Can you work these out from the model? Positions are in its coordinate system, mm. Face numbers are marked on the shaded views. A direction names the side the tool comes from. Coordinates: 2 decimals unless noted, no trailing zeros. Write each loop counter-clockwise with the first axis right and the second up, starting at its lowest first coordinate (ties: lowest second). Pieces come first, ordered by that corner, then holes. Notation, with made-up numbers: M 0,25.25 L 11,25.25 A6 ccw 11,29.25 Z; hole C -0.5,-2 d3. An arc over 180 degrees is marked long. Use one line per item in the form item = value. Start each with the question number.
Autodesk Fusion 360 part; units mm, degrees
sketch "Sketch1" plane through (0, 0, 0) normal (1, 0, 0) x (0, 1, 0)
  line L0 (0, 0) -> (-25.4, 0)
  line L1 (-25.4, 0) -> (-25.4, 43.18)
  line L2 (-25.4, 43.18) -> (-19.05, 43.18)
  line L3 (0, 0) -> (0, 43.18)
  line L4 (0, 43.18) -> (-6.35, 43.18)
  line L5 (-6.35, 43.18) -> (-6.35, 17.78)
  line L6 (-19.05, 43.18) -> (-19.05, 17.7768)
  line L7 (-19.05, 17.7768) -> (-6.35, 17.78)
  circle A0 centre (-12.7, 7.62) radius 5.08
  dimension "d1" = 25.4
  dimension "d2" = 43.18
  dimension "d3" = 6.35
  dimension "d5" = 25.4
  dimension "d6" = 10.16
  dimension "d7" = 12.7
  dimension "d8" = 7.62
  dimension "d10" = 6.35
  dimension "d11" = 12.7
  dimension "d12" = 43.18
extrude "Extrude1" add sketch "Sketch1" along normal blind 25.4
sketch "Sketch2" plane through (25.4, 0, 0) normal (1, 0, 0) x (0, 1, 0)
  circle A0 centre (-12.7, 7.62) radius 5.08
  line L0 (0, 0) -> (0, 43.18)
  line L1 (0, 43.18) -> (-6.35, 43.18)
  line L2 (-6.35, 43.18) -> (-6.35, 17.78)
  line L3 (-6.35, 17.78) -> (-19.05, 17.7768)
  line L4 (-19.05, 17.7768) -> (-19.05, 43.18)
  line L5 (-19.05, 43.18) -> (-25.4, 43.18)
  line L6 (-25.4, 43.18) -> (-25.4, 0)
  line L7 (-25.4, 0) -> (0, 0)
  line L8 (-25.4, 0) -> (0, 0)
  line L9 (0, 0) -> (0, 16.51)
  line L10 (0, 16.51) -> (-25.4, 16.51)
  line L11 (-25.4, 16.51) -> (-25.4, 0)
  dimension "d28" = 16.51
extrude "Extrude2" cut sketch "Sketch2" against normal blind 6.3551 contours L0 L6 L7 L8 L9 L10 L11
sketch "Sketch3" plane through (0, 0, 0) normal (-1, 0, 0) x (0, -1, 0)
  circle A0 centre (12.7, 7.62) radius 5.08
  line L0 (0, 43.18) -> (0, 0)
  line L1 (0, 0) -> (25.4, 0)
  line L2 (25.4, 0) -> (25.4, 43.18)
  line L3 (25.4, 43.18) -> (19.05, 43.18)
  line L4 (19.05, 43.18) -> (19.05, 17.7768)
  line L5 (19.05, 17.7768) -> (6.35, 17.78)
  line L6 (6.35, 17.78) -> (6.35, 43.18)
  line L7 (6.35, 43.18) -> (0, 43.18)
  line L8 (0, 0) -> (25.4, 0)
  line L9 (25.4, 0) -> (25.4, 16.51)
  line L10 (25.4, 16.51) -> (0, 16.51)
  line L11 (0, 16.51) -> (0, 0)
  dimension "d29" = 16.51
extrude "Extrude3" cut sketch "Sketch3" against normal blind 6.3551 contours L0 L1 L2 L8 L9 L10 L11
sketch "Sketch4" plane through (0, -25.4, 0) normal (0, -1, 0) x (1, 0, 0)
  line L0 (6.3551, 16.51) -> (6.3551, 0)
  line L1 (6.3551, 0) -> (19.0449, 0)
  line L2 (19.0449, 0) -> (19.0449, 16.51)
  line L3 (19.0449, 16.51) -> (25.4, 16.51)
  line L4 (25.4, 16.51) -> (25.4, 43.18)
  line L5 (25.4, 43.18) -> (0, 43.18)
  line L6 (0, 43.18) -> (0, 16.51)
  line L7 (0, 16.51) -> (6.3551, 16.51)
  line L8 (0, 43.18) -> (25.4422, 43.18)
  line L9 (25.4422, 43.18) -> (25.4422, 17.78)
  line L10 (25.4422, 17.78) -> (0, 17.78)
  line L11 (0, 17.78) -> (0, 43.18)
  circle A0 centre (12.7, 25.4) radius 2.54
  circle A1 centre (12.7, 35.56) radius 5.08
  dimension "d19" = 25.4
  dimension "d20" = 5.08
  dimension "d22" = 12.7
  dimension "d23" = 10.16
  dimension "d24" = 7.62
  dimension "d25" = 12.7
  dimension "d47" = 10.16
extrude "Extrude4" cut sketch "Sketch4" against normal blind 40.64 contours A0 | A1
fillet "Fillet1" radius 12.7 2 edges at (12.7, -25.4, 0) (12.7, 0, 0)
chamfer "Chamfer1" distance 6.0452 angle 50 2 edges at (25.4, -22.225, 43.18) (25.4, -3.175, 43.18) measured on face at (8.4667, -23.2833, 43.18) measured on face at (8.4667, -2.1167, 43.18)
chamfer "Chamfer2" distance 4.572 angle 20 1 edges at (0, -3.175, 43.18) measured on face at (12.9032, -2.1167, 43.18)
chamfer "Chamfer3" distance 4.572 angle 20 1 edges at (0, -22.225, 43.18) measured on face at (12.9032, -23.2833, 43.18)
sketch "Sketch5" plane through (0, -25.4, 0) normal (0, -1, 0) x (1, 0, 0)
  line L0 (4.572, 43.18) -> (0, 41.5159)
  line L1 (0, 41.5159) -> (0, 16.51)
  line L2 (0, 16.51) -> (6.3551, 16.51)
  line L3 (6.3551, 16.51) -> (6.3551, 12.7)
  line L4 (6.3551, 12.7) -> (19.0449, 12.7)
  line L5 (19.0449, 12.7) -> (19.0449, 16.51)
  line L6 (19.0449, 16.51) -> (25.4, 16.51)
  line L7 (25.4, 16.51) -> (25.4, 35.9756)
  line L8 (25.4, 35.9756) -> (19.3548, 43.18)
  line L9 (19.3548, 43.18) -> (4.572, 43.18)
  circle A0 centre (12.7, 35.56) radius 5.08
  circle A1 centre (12.7, 25.4) radius 2.54
  line L10 (0, 41.5159) -> (-2.6255, 40.5603)
  line L11 (-2.6255, 40.5603) -> (0, 38.3573)
  dimension "d38" = 2.794
  dimension "d39" = 60
extrude "Extrude5" add sketch "Sketch5" against normal blind 6.35 contours L1 L10 L11
sketch "Sketch6" plane through (0, 0, 0) normal (0, 1, 0) x (-1, 0, 0)
  line L0 (0, 41.5159) -> (-4.572, 43.18)
  line L1 (-4.572, 43.18) -> (-19.3548, 43.18)
  line L2 (-19.3548, 43.18) -> (-25.4, 35.9756)
  line L3 (-25.4, 35.9756) -> (-25.4, 16.51)
  line L4 (-25.4, 16.51) -> (-19.0449, 16.51)
  line L5 (-19.0449, 16.51) -> (-19.0449, 12.7)
  line L6 (-19.0449, 12.7) -> (-6.3551, 12.7)
  line L7 (-6.3551, 12.7) -> (-6.3551, 16.51)
  line L8 (-6.3551, 16.51) -> (0, 16.51)
  line L9 (0, 16.51) -> (0, 41.5159)
  circle A0 centre (-12.7, 25.4) radius 2.54
  circle A1 centre (-12.7, 35.56) radius 5.08
  line L10 (0, 41.5159) -> (2.6255, 40.5603)
  line L11 (2.6255, 40.5603) -> (0, 38.354)
  line L12 (0, 38.354) -> (0, 41.5159)
  dimension "d42" = 2.794
extrude "Extrude6" add sketch "Sketch6" against normal blind 6.35 contours L9 L10 L11 L12
fillet "Fillet2" radius 1.27 2 edges at (19.3548, -22.225, 43.18) (19.3548, -3.175, 43.18)
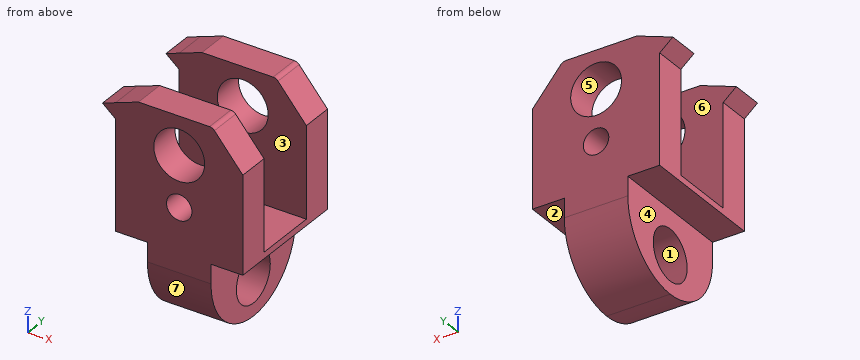
1) Suppose I cut it at A-A on x = 12.7. State how many separate pieces and enclosed holes the cut face has, and give its area (3 significant figures).
2) Suppose I cut it at D-D on z = 7.62. Please give me the cut outline in (x, y).
3) Which directions (+Z, -Z, +X, -X, +Y, -Y) give clear straight access to the entire face, cutting with the end or side of a thin tool? Please do the marked faces 1, 2, 3 and 4.
4) Will these pins go through, and if not, where does the flat tip stop? pin 1 Ø10 at (y, z) = (-8, 9.5) entering from +X; pin 2 Ø9 at (x, z) = (12.7, 35.56) entering from -Y; pin 3 Ø3 at (x, y) = (19.5, -10) entering from +Z; pin 4 Ø5 at (y, z) = (-10.5, 16) entering from -X.
5) Suppose I cut it at B-B on y = -4. Please give me the cut outline in (x, z).
6) If we mould it in two halves opening along Y, with no side actions, what happens to the marked faces 5, 6 and 7? For each: +Y half, -Y half, draft (parallel to the pull), parting line (faces both ways), or undercut.
7) Please list where these lines run through material, in increasing order: line 1 (Y direction, x = 21.25, z = 37); line 2 (Z direction, x = 12.7, y = -20.5); line 3 (Z direction, x = 12.7, y = -3.25).
Computed values:
q1.separate_pieces = 5
q1.enclosed_holes = 1
q1.area = 430 mm²
q2.outline = M 6.36,-24.34 L 19.04,-24.34 L 19.04,-17.78 L 6.36,-17.78 Z; M 6.36,-7.62 L 19.04,-7.62 L 19.04,-1.06 L 6.36,-1.06 Z
q3.face_1 = +X, -X
q3.face_2 = -Z, +X, +Y, -Y
q3.face_3 = +Z, +X, -X
q3.face_4 = -Z, -X, +Y, -Y
q4.pin_1 = 19.04
q4.pin_2 = through
q4.pin_3 = 17.78
q4.pin_4 = 0
q5.outline = M -2.63,40.56 L 0,38.35 L 0,16.51 L 6.36,16.51 L 6.36,3.45 L 19.04,3.45 L 19.04,16.51 L 25.4,16.51 L 25.4,35.98 L 19.74,42.73 A1.27 ccw 18.76,43.18 L 4.57,43.18 L 0,41.52 Z; hole C 12.7,35.56 d10.16; hole C 12.7,25.4 d5.08
q6.face_5 = draft
q6.face_6 = undercut
q6.face_7 = -Y half
q7.line_1 = -25.4 to -19.05, -6.35 to 0
q7.line_2 = 2.68 to 22.86, 27.94 to 30.48, 40.64 to 43.18
q7.line_3 = 4.21 to 22.86, 27.94 to 30.48, 40.64 to 43.18
